```python
from build123d import *

# Parameters (mm, degrees)
SKETCH_1_R      = 1.5
EXTRUDE_1_DEPTH = 3


with BuildPart() as part:
    # 草圖1 → 填料-伸長1 (new body)
    with BuildSketch(Plane(origin=(0, 3, 0), x_dir=(1, 0, 0), z_dir=(0, 1, 0))):
        with BuildLine():
            Line((-46, 43), (-46, -43))
            ThreePointArc((-46, -43), (-45.121320344, -45.121320344), (-43, -46))
            Line((-43, -46), (43, -46))
            ThreePointArc((43, -46), (45.121320344, -45.121320344), (46, -43))
            Line((46, -43), (46, 43))
            ThreePointArc((46, 43), (45.121320344, 45.121320344), (43, 46))
            Line((43, 46), (-43, 46))
            ThreePointArc((-43, 46), (-45.121320344, 45.121320344), (-46, 43))
        make_face()
        with Locations((41.25, -41.25)):
            Circle(SKETCH_1_R, mode=Mode.SUBTRACT)
        with Locations((-41.25, 41.25)):
            Circle(SKETCH_1_R, mode=Mode.SUBTRACT)
        with Locations((41.25, 41.25)):
            Circle(SKETCH_1_R, mode=Mode.SUBTRACT)
        with Locations((-41.25, -41.25)):
            Circle(SKETCH_1_R, mode=Mode.SUBTRACT)
        with BuildLine():
            Line((-31.378679656, 26.628679656), (-6.871320344, 2.121320344))
            ThreePointArc((-6.871320344, 2.121320344), (-5.992640687, 0), (-6.871320344, -2.121320344))
            Line((-6.871320344, -2.121320344), (-31.378679656, -26.628679656))
            ThreePointArc((-31.378679656, -26.628679656), (-34.648050297, -27.27899791), (-36.5, -24.507359313))
            Line((-36.5, -24.507359313), (-36.5, 24.507359313))
            ThreePointArc((-36.5, 24.507359313), (-34.648050297, 27.27899791), (-31.378679656, 26.628679656))
        make_face(mode=Mode.SUBTRACT)
        with BuildLine():
            Line((24.507359313, -36.5), (-24.507359313, -36.5))
            ThreePointArc((-24.507359313, -36.5), (-27.27899791, -34.648050297), (-26.628679656, -31.378679656))
            Line((-26.628679656, -31.378679656), (-2.121320344, -6.871320344))
            ThreePointArc((-2.121320344, -6.871320344), (0, -5.992640687), (2.121320344, -6.871320344))
            Line((2.121320344, -6.871320344), (26.628679656, -31.378679656))
            ThreePointArc((26.628679656, -31.378679656), (27.27899791, -34.648050297), (24.507359313, -36.5))
        make_face(mode=Mode.SUBTRACT)
        with BuildLine():
            Line((-24.507359313, 36.5), (24.507359313, 36.5))
            ThreePointArc((24.507359313, 36.5), (27.27899791, 34.648050297), (26.628679656, 31.378679656))
            Line((26.628679656, 31.378679656), (2.121320344, 6.871320344))
            ThreePointArc((2.121320344, 6.871320344), (0, 5.992640687), (-2.121320344, 6.871320344))
            Line((-2.121320344, 6.871320344), (-26.628679656, 31.378679656))
            ThreePointArc((-26.628679656, 31.378679656), (-27.27899791, 34.648050297), (-24.507359313, 36.5))
        make_face(mode=Mode.SUBTRACT)
        with BuildLine():
            Line((36.5, 24.507359313), (36.5, -24.507359313))
            ThreePointArc((36.5, -24.507359313), (34.648050297, -27.27899791), (31.378679656, -26.628679656))
            Line((31.378679656, -26.628679656), (6.871320344, -2.121320344))
            ThreePointArc((6.871320344, -2.121320344), (5.992640687, 0), (6.871320344, 2.121320344))
            Line((6.871320344, 2.121320344), (31.378679656, 26.628679656))
            ThreePointArc((31.378679656, 26.628679656), (34.648050297, 27.27899791), (36.5, 24.507359313))
        make_face(mode=Mode.SUBTRACT)
    extrude(amount=-EXTRUDE_1_DEPTH)


solid = part.part
```
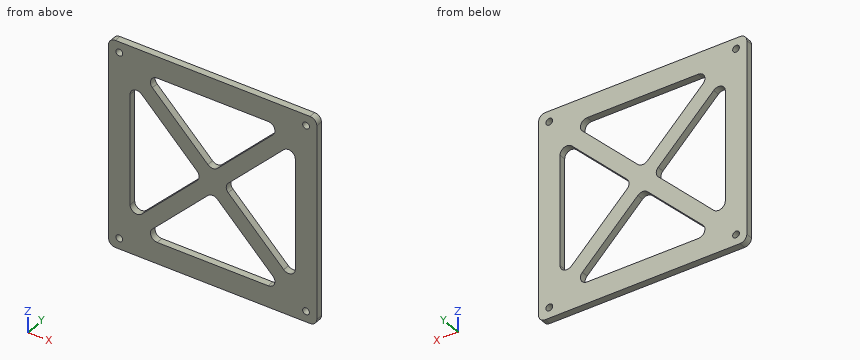
Here's how the part is built. I have some questions about the finished solid (model axes, mm). Give positions to 0.01 mm unless a question says otherwise; leave off trailing zeros. Order: outer loops, then holes, each group sorted by start corner. A loop starts at its lowest first (then second) coordinate and runs counter-clockwise, first axis right, second up. Notation, with made-up numbers: M 3,66 L 60,66 A22 ccw 60,94 Z; hole C -6,57.25 d1. An arc over 180 degrees is marked long. Use a Markdown table: item, result. Add a question column.
1. Suppose I cut it at B-B (z = 41.25). List the corners of the cut face in (x, y) for me.
2. For pin 1 Ø1.8 at (x, z) = (41.25, 41.25) entering from +Y, with a flat end and sliding along its axis, tell me the tip position at first contact or that it passes through.
3. Suppose I cut it at D-D (x = -18). List the corners of the cut face in (y, z) for me, and give its area (3 significant figures).
4. Suppose I cut it at C-C (z = 17). List the corners of the cut face in (x, y) for me.
5. Suppose I cut it at A-A (x = -41.25). List the corners of the cut face in (y, z) for me, and give its area (3 significant figures).
6. I need wall thicknesses on probe 1 along X at (y, z) = (2, 41.25); probe 2 along Z at (x, y) = (-2, 0.65). Which ranges of each line are inside material? Lowest first, please. Write a range as from..to.
Results list:
| question | item | result |
|---|---|---|
| 1 | outline | M -46,0 L -42.75,0 L -42.75,3 L -46,3 Z; M -39.75,0 L 39.75,0 L 39.75,3 L -39.75,3 Z; M 42.75,0 L 46,0 L 46,3 L 42.75,3 Z |
| 2 | pin 1 | passes through |
| 3 | outline | M 0,-46 L 3,-46 L 3,-36.5 L 0,-36.5 Z; M 0,-22.75 L 3,-22.75 L 3,-13.25 L 0,-13.25 Z; M 0,13.25 L 3,13.25 L 3,22.75 L 0,22.75 Z; M 0,36.5 L 3,36.5 L 3,46 L 0,46 Z |
| 3 | area | 114 mm² |
| 4 | outline | M -46,0 L -36.5,0 L -36.5,3 L -46,3 Z; M -21.75,0 L -12.25,0 L -12.25,3 L -21.75,3 Z; M 12.25,0 L 21.75,0 L 21.75,3 L 12.25,3 Z; M 36.5,0 L 46,0 L 46,3 L 36.5,3 Z |
| 5 | outline | M 0,-46 L 3,-46 L 3,-42.75 L 0,-42.75 Z; M 0,-39.75 L 3,-39.75 L 3,39.75 L 0,39.75 Z; M 0,42.75 L 3,42.75 L 3,46 L 0,46 Z |
| 5 | area | 258 mm² |
| 6 | probe 1 | x = -46..-42.75, -39.75..39.75, 42.75..46 |
| 6 | probe 2 | z = -46..-36.5, -6.76..6.76, 36.5..46 |
